Study the drawing (mm; zero at the part's minimum x, y, z) and answer. A direction names the side the tool comes from. Coordinates: 2 decimals unless noted, no trailing zeros. Loops run counter-clockwise (first coordinate to the right, second up) from the corner with the lowest first, then second, coordinate; pieces in that order, holes last. Notation, with made-up numbers: (88.25, -11) -> (121.25, -11) arc R26 cw to (121.25, 4) -> close; hole circle Ø7 at (73, 1.25). An arc over 180 degrees is marked (long way). Answer in a Markdown table with one row per item.
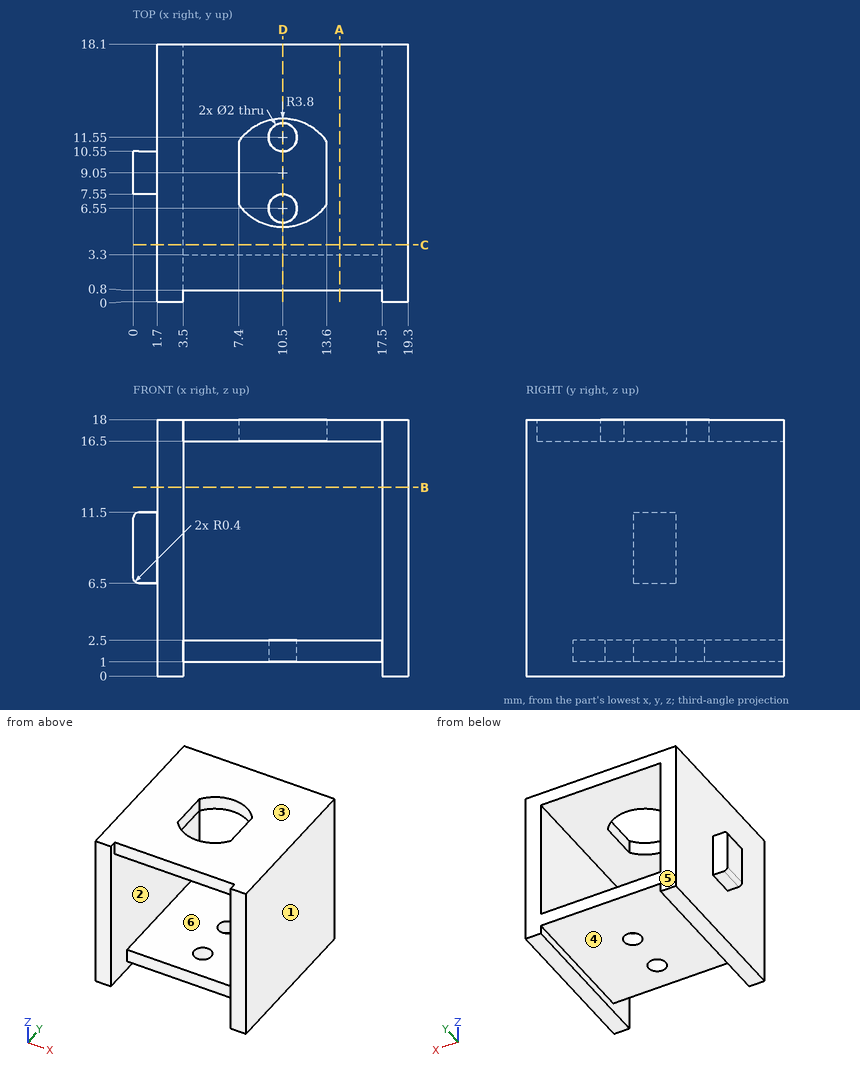
1. A tool of negligible diameter and unlimited length cuts with its end or side. For the marked faces 4, 5 and 6, from which of +Z, -Z, +X, -X, +Y, -Y can it reach the whole face along a straight path? Write none if from no direction.
A:
| item | result |
|---|---|
| face 4 | -Z, +Y, -Y |
| face 5 | +Z, -Z, +X, -X, +Y |
| face 6 | +Y, -Y |
2. Given pin 1 Ø2.5 at (x, y) = (10.5, 6.55) entering from -Z; pin 2 Ø5 at (x, z) = (9, 6) entering from +Y; pin 3 Ø0.5 at (x, z) = (1, 8) entering from -Y; pin 4 Ø1.2 at (y, z) = (8.5, 17.5) entering from -X, each flat-ended and moving along its own axis, determine where each tip first touches the part or whether it passes through.
A:
| item | result |
|---|---|
| pin 1 | stops at z = 1 |
| pin 2 | passes through |
| pin 3 | stops at y = 7.55 |
| pin 4 | stops at x = 1.7 |
3. A cutting plane is placed at A-A on x = 14.5. Give the vertices of the cut face in (y, z).
A:
| item | result |
|---|---|
| outline | (0.8, 16.5) -> (18.1, 16.5) -> (18.1, 18) -> (0.8, 18) -> close; (3.3, 1) -> (18.1, 1) -> (18.1, 2.5) -> (3.3, 2.5) -> close |
4. Find the intervals of material crossed by probe 1 along Z at (x, y) = (16.5, 14.25); probe 2 along X at (y, z) = (3.75, 5.5); probe 3 along Y at (x, z) = (10.5, 1.55), in increasing order.
A:
| item | result |
|---|---|
| probe 1 | z = 1 to 2.5, 16.5 to 18 |
| probe 2 | x = 1.7 to 3.5, 17.5 to 19.3 |
| probe 3 | y = 3.3 to 5.55, 7.55 to 10.55, 12.55 to 18.1 |
5. A cutting plane is placed at C-C on y = 4. Give the vertices of the cut face in (x, z), and give its area (3 significant figures).
A:
| item | result |
|---|---|
| outline | (1.7, 0) -> (3.5, 0) -> (3.5, 1) -> (17.5, 1) -> (17.5, 0) -> (19.3, 0) -> (19.3, 18) -> (1.7, 18) -> close; hole (3.5, 2.5) -> (17.5, 2.5) -> (17.5, 16.5) -> (3.5, 16.5) -> close |
| area | 107 mm2 |
6. The mould has two halves that part along X. Classify the marked faces 1, 2 and 3: pulls with the +X half, pulls with the -X half, needs draft (parallel to the pull), parting line crosses it, or undercut.
A:
| item | result |
|---|---|
| face 1 | pulls with the +X half |
| face 2 | undercut |
| face 3 | needs draft |
7. A cutting plane is placed at D-D on x = 10.5. Give the vertices of the cut face in (y, z).
A:
| item | result |
|---|---|
| outline | (0.8, 16.5) -> (5.25, 16.5) -> (5.25, 18) -> (0.8, 18) -> close; (3.3, 1) -> (5.55, 1) -> (5.55, 2.5) -> (3.3, 2.5) -> close; (7.55, 1) -> (10.55, 1) -> (10.55, 2.5) -> (7.55, 2.5) -> close; (12.55, 1) -> (18.1, 1) -> (18.1, 2.5) -> (12.55, 2.5) -> close; (12.85, 16.5) -> (18.1, 16.5) -> (18.1, 18) -> (12.85, 18) -> close |
8. A cutting plane is placed at B-B on z = 13.25. Give the vertices of the cut face in (x, y), and give its area (3 significant figures).
A:
| item | result |
|---|---|
| outline | (1.7, 0) -> (3.5, 0) -> (3.5, 18.1) -> (1.7, 18.1) -> close; (17.5, 0) -> (19.3, 0) -> (19.3, 18.1) -> (17.5, 18.1) -> close |
| area | 65.2 mm2 |
